from build123d import *

# Parameters (mm, degrees)
SKETCH_R             = 7
SKETCH_R_2           = 6.5
PAD_DEPTH            = 120
REVOLUTION_FACE7_R   = 7
REVOLUTION_FACE7_R_2 = 6.5
POCKET_DEPTH         = 8.5
SKETCH003_W          = 5
SKETCH003_H          = 35
POCKET001_DEPTH      = 5


with BuildPart() as part:
    # Sketch → Pad (new body)
    with BuildSketch(Plane.XY):
        Circle(SKETCH_R)
        Circle(SKETCH_R_2, mode=Mode.SUBTRACT)
    extrude(amount=PAD_DEPTH)

    # Sketch001 → Revolution (revolve)
    with BuildSketch(Plane.XZ):
        Polygon((0.917134, 0), (7, 10.535833), (7, 9.41), (1.567134, 0), align=None)
    revolve(axis=Axis((0, 0, 0), (0, 0, 1)))

    # Revolution Face7 → Pocket (cut)
    with BuildSketch(Plane(origin=(0, 0, 0), x_dir=(0, -1, 0), z_dir=(0, 0, -1))):
        Circle(REVOLUTION_FACE7_R)
        Circle(REVOLUTION_FACE7_R_2, mode=Mode.SUBTRACT)
    extrude(amount=-POCKET_DEPTH, mode=Mode.SUBTRACT)

    # Sketch003 → Pocket001 (cut)
    with BuildSketch(Plane.XZ):
        with Locations((4.91, 77.5)):
            Rectangle(SKETCH003_W, SKETCH003_H)
    extrude(amount=-POCKET001_DEPTH, mode=Mode.SUBTRACT)


solid = part.part
Source: CAD feature listing. Evaluate the final solid. Frame: model axes, mm. Coordinates: 2 decimals unless noted, no trailing zeros. Loops run counter-clockwise (first coordinate to the right, second up) from the corner with the lowest first, then second, coordinate; pieces in that order, holes last. Notation, with made-up numbers: (37, 40) - (62, 40) arc R26 cw to (62, 73) - close; hole circle Ø1 at (-11.5, 74.25). An arc over 180 degrees is marked (long way). One line per item, written item: value. Start each with the question number.
1. Section A-A (z = 59). Return the cut outline in (x, y).
2. Contact query for flat-ended pins moving along their axis: P1, Ø5, axis at x = -4.5, z = 64.5, coming from the +Y side; P2, Ø2, axis at y = 2, z = 55, coming from the -X side; P3, Ø1.5, axis at x = 3, y = 3, coming from the +Z side; P4, Ø0.9, axis at x = 6, y = 1.5, coming from the +Z side. Output: stop coordinate, or through.
3. Mould query, pull axis Y, two halves, no side actions, for faces 1 (the flat face through (1, -1, 0)), 2 (the conical face through (-0.63, -2.83, 2.31)), 3 (the conical face through (1.35, 2.11, 2.75)), 4 (the cylindrical face through (-5.158, -3.955, 64.063)). Classes: pulls with the +Y half, pulls with the -Y half, needs draft (parallel to the pull), parting line crosses it, or undercut.
4. Section B-B (z = 73). Return the cut outline in (x, y), and give its area (3 significant figures).
5. Ray query, L1, parallel to Y at x = -0.5, z = 24.5; L2, parallel to Y at x = -1.5, z = 41; L3, parallel to X at y = -4.5, z = 49. Return the intervals inside material, ascending.
Verdict:
1. outline: circle Ø14 at (0, 0); hole circle Ø13 at (0, 0)
2. P1: stops at y = 6.71
2. P2: stops at x = -6.93
2. P3: stops at z = 7.06
2. P4: stops at z = 120
3. face 1: needs draft
3. face 2: parting line crosses it
3. face 3: undercut
3. face 4: undercut
4. outline: (4.15, 5) - (4.9, 5) arc R7 ccw (long way) to (7, 0) - (6.5, 0) arc R6.5 cw (long way) to start
4. area: 18.4 mm2
5. L1: y = -6.98 to -6.48, 6.48 to 6.98
5. L2: y = -6.84 to -6.32, 6.32 to 6.84
5. L3: x = -5.36 to -4.69, 4.69 to 5.36
